```python
from build123d import *

# Parameters (mm, degrees)
F1_W      = 603.25
F1_H      = 234.95
F2_DEPTH  = 12.065
F3_W      = 12.065
F3_H      = 234.95
F4_DEPTH  = 6.0325
F5_W      = 12.065
F5_H      = 234.95
F6_DEPTH  = 6.0325
F7_W      = 12.065
F7_H      = 234.95
F8_DEPTH  = 6.0325
F9_W      = 12.065
F9_H      = 234.95
F10_DEPTH = 6.0325
F11_W     = 203.2
F11_H     = 12.065
F14_DEPTH = 6.0325
F12_W     = 148.59
F12_H     = 12.065
F15_DEPTH = 6.0325
F13_W     = 203.2
F13_H     = 12.065
F16_DEPTH = 6.0325
F17_W     = 12.065
F17_H     = 31.75
F18_DEPTH = 6.0325
F19_W     = 12.065
F19_H     = 31.75
F20_DEPTH = 6.0325
F21_W     = 107.95
F21_H     = 139.7
F22_DEPTH = 12.065


# Not quite as in the source:
# - a variable given as a bare number and used for a length is read in inches; the dataset says mm whatever the document's units were


with BuildPart() as f2:
    # F1 (on Top) → F2 (new body)
    with BuildSketch(Plane.XY):
        Rectangle(F1_W, F1_H)
    extrude(amount=F2_DEPTH)

    # F3 (on face) → F4 (cut)
    with BuildSketch(Plane(origin=(0, 0, 0), x_dir=(1, 0, 0), z_dir=(0, 0, -1))):
        with Locations((-295.5925, 0)):
            Rectangle(F3_W, F3_H)
    extrude(amount=-F4_DEPTH, mode=Mode.SUBTRACT)

    # F5 (on face) → F6 (cut)
    with BuildSketch(Plane(origin=(0, 0, 0), x_dir=(1, 0, 0), z_dir=(0, 0, -1))):
        with Locations((295.5925, 0)):
            Rectangle(F5_W, F5_H)
    extrude(amount=-F6_DEPTH, mode=Mode.SUBTRACT)

    # F7 (on face) → F8 (cut)
    with BuildSketch(Plane(origin=(0, 0, 0), x_dir=(1, 0, 0), z_dir=(0, 0, -1))):
        with Locations((80.3275, 0)):
            Rectangle(F7_W, F7_H)
    extrude(amount=-F8_DEPTH, mode=Mode.SUBTRACT)

    # F9 (on face) → F10 (cut)
    with BuildSketch(Plane(origin=(0, 0, 0), x_dir=(1, 0, 0), z_dir=(0, 0, -1))):
        with Locations((-80.3275, 0)):
            Rectangle(F9_W, F9_H)
    extrude(amount=-F10_DEPTH, mode=Mode.SUBTRACT)

    # F11 (on face) → F14 (cut)
    with BuildSketch(Plane(origin=(0, 0, 0), x_dir=(1, 0, 0), z_dir=(0, 0, -1))):
        with Locations((187.96, -111.4425)):
            Rectangle(F11_W, F11_H)
    extrude(amount=-F14_DEPTH, mode=Mode.SUBTRACT)

    # F12 (on face) → F15 (cut)
    with BuildSketch(Plane(origin=(0, 0, 0), x_dir=(1, 0, 0), z_dir=(0, 0, -1))):
        with Locations((0, -111.4425)):
            Rectangle(F12_W, F12_H)
    extrude(amount=-F15_DEPTH, mode=Mode.SUBTRACT)

    # F13 (on face) → F16 (cut)
    with BuildSketch(Plane(origin=(0, 0, 0), x_dir=(1, 0, 0), z_dir=(0, 0, -1))):
        with Locations((-187.96, -111.4425)):
            Rectangle(F13_W, F13_H)
    extrude(amount=-F16_DEPTH, mode=Mode.SUBTRACT)

    # F17 (on face) → F18 (join)
    with BuildSketch(Plane(origin=(0, 0, 6.0325), x_dir=(1, 0, 0), z_dir=(0, 0, -1))):
        with Locations((80.3275, 101.6)):
            Rectangle(F17_W, F17_H)
    extrude(amount=F18_DEPTH)

    # F19 (on face) → F20 (join)
    with BuildSketch(Plane(origin=(0, 0, 6.0325), x_dir=(1, 0, 0), z_dir=(0, 0, -1))):
        with Locations((-80.3275, 101.6)):
            Rectangle(F19_W, F19_H)
    extrude(amount=F20_DEPTH)

    # F21 (on face) → F22 (cut)
    with BuildSketch(Plane.XY.offset(12.065)):
        Rectangle(F21_W, F21_H)
    extrude(amount=-F22_DEPTH, mode=Mode.SUBTRACT)


solid = f2.part
```
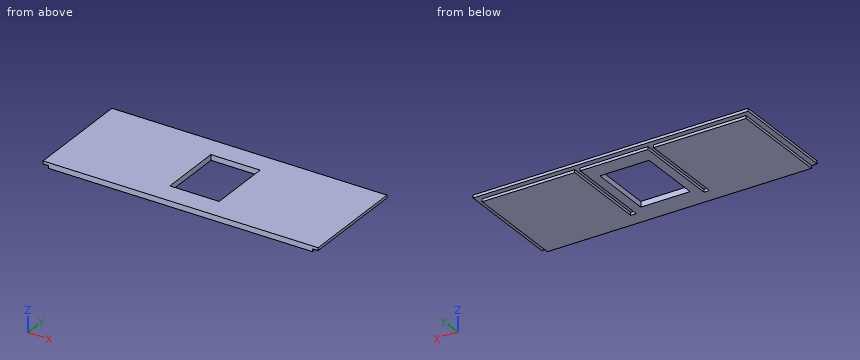
For this review, take the finished solid that the model builds, in its own axes (mm). Coordinates: 2 decimals unless noted, no trailing zeros. Write each loop counter-clockwise with the first axis right and the second up, starting at its lowest first coordinate (ties: lowest second). Pieces come first, ordered by that corner, then holes. Notation, with made-up numbers: (39.5, 72.5) - (84.5, 72.5) arc R28 ccw to (84.5, 99.5) - close; hole circle Ø3 at (-20.75, 9). An arc over 180 degrees is marked (long way). Put each result on its own line as item: value.
1. Wall thickness on probe 1 along X at (y, z) = (68, 6) (3 decimals); probe 2 along X at (y, z) = (99, 1.75) (3 decimals); probe 3 along Y at (x, z) = (3, 9.5) (3 decimals): over which ranges is each line inside the solid? List them lowest first.
Values found:
probe 1: -289.56 to -86.36, -74.295 to -53.975, 53.975 to 74.295, 86.36 to 289.56
probe 2: -289.56 to -86.36, -74.295 to 74.295, 86.36 to 289.56
probe 3: -117.475 to -69.85, 69.85 to 117.475
2. For pin 1 (3 mm diameter, centred on x = 215.5, z = 3.5, fed in from +Y); pin 2 (6.5 mm diameter, centred on x = -4.5, z = 3, fed in from +Y) (3 decimals); pin 3 (3 mm diameter, centred on x = 79.5, z = 4, fed in from +Y) (3 decimals); pin 4 (5 mm diameter, centred on y = 13, z = 2, fed in from -X), all flat-tipped, find the tip position at first contact; note any pin that passes through.
Values found:
pin 1: y = 105.41
pin 2: y = 117.475
pin 3: y = -85.725
pin 4: x = -289.56
3. Add section A-A, the plane y = 0. Give the boundary of the cut face in (x, z) (1 decimal).
Values found:
outline: (-301.6, 6) - (-289.6, 6) - (-289.6, 0) - (-86.4, 0) - (-86.4, 6) - (-74.3, 6) - (-74.3, 0) - (-54, 0) - (-54, 12.1) - (-301.6, 12.1) - close; (54, 0) - (74.3, 0) - (74.3, 6) - (86.4, 6) - (86.4, 0) - (289.6, 0) - (289.6, 6) - (301.6, 6) - (301.6, 12.1) - (54, 12.1) - close
4. Add section D-D, the plane x = 176. Give the boundary of the cut face in (y, z) (1 decimal), then the cut area to 3 significant figures.
Values found:
outline: (-117.5, 0) - (105.4, 0) - (105.4, 6) - (117.5, 6) - (117.5, 12.1) - (-117.5, 12.1) - close
area: 2,760 mm²
5. Add section B-B, the plane z = 4. Give the boundary of the cut face in (x, y) (3 decimals).
Values found:
outline: (-289.56, -117.475) - (289.56, -117.475) - (289.56, 105.41) - (86.36, 105.41) - (86.36, -85.725) - (74.295, -85.725) - (74.295, 105.41) - (-74.295, 105.41) - (-74.295, -85.725) - (-86.36, -85.725) - (-86.36, 105.41) - (-289.56, 105.41) - close; hole (-53.975, -69.85) - (53.975, -69.85) - (53.975, 69.85) - (-53.975, 69.85) - close
